Check sheet for the modelled part. Datum: model origin and axes. Units: mm. A direction names the side the tool comes from. Coordinates: 2 decimals unless noted, no trailing zeros. Order: outer loops, then holes, each group sorted by start corner. A loop starts at its lowest first (then second) coordinate and runs counter-clockwise, first axis right, second up.
from build123d import *

# Parameters (mm, degrees)
SKETCH2_R                           = 6.35
BOSS_EXTRUDE1_DEPTH                 = 12.7
FILLET3_R                           = 11.43
F_7_32_0_21875_DIAMETER_HOLE1_D     = 5.55625
F_7_32_0_21875_DIAMETER_HOLE1_DEPTH = 36.430734093
F_7_32_0_21875_DIAMETER_HOLE1_TIP   = 1.669265907


with BuildPart() as part:
    # Sketch2 → Boss-Extrude1 (new body)
    with BuildSketch(Plane.XY):
        Polygon((0, 0), (40.64, 0), (40.64, -10.16), (25.4, -10.16), (25.4, -22.86), (0, -22.86), align=None)
        with Locations((12.7, -11.43)):
            Circle(SKETCH2_R, mode=Mode.SUBTRACT)
    extrude(amount=BOSS_EXTRUDE1_DEPTH)

    # Fillet3
    fillet3_edges = [part.edges().sort_by_distance(p)[0] for p in [
        (0, -22.86, 6.35),
        (0, 0, 6.35),
    ]]
    fillet(fillet3_edges, radius=FILLET3_R - 0.0001)  # a hair under: the kernel refuses the full size

    # 7/32 (0.21875) Diameter Hole1
    with Locations(Plane(origin=(33.02, 0, 6.35), x_dir=(0, 0, 1), z_dir=(0, 1, 0))):
        with Locations((0, 0)):
            Hole(F_7_32_0_21875_DIAMETER_HOLE1_D / 2, depth=F_7_32_0_21875_DIAMETER_HOLE1_DEPTH)
            with Locations((0, 0, -(F_7_32_0_21875_DIAMETER_HOLE1_DEPTH + F_7_32_0_21875_DIAMETER_HOLE1_TIP / 2))):  # 118° drill point
                Cone(0, F_7_32_0_21875_DIAMETER_HOLE1_D / 2, F_7_32_0_21875_DIAMETER_HOLE1_TIP, mode=Mode.SUBTRACT)


solid = part.part
(1) Cross-section at A-A (x = 12.7). Enter the section's corners in (y, z).
Filled in:
outline: (-22.86, 0) - (-17.78, 0) - (-17.78, 12.7) - (-22.86, 12.7) - close; (-5.08, 0) - (0, 0) - (0, 12.7) - (-5.08, 12.7) - close
(2) Go/stop test with flat-tipped pins: P1, Ø4.5, axis at x = 33.02, z = 6.35, coming from the +Y side; P2, Ø1, axis at y = -19, z = 9.5, coming from the -X side; P3, Ø4, axis at x = 35, z = 7.5, coming from the -Y side; P4, Ø6, axis at y = -16, z = 9, coming from the -X side. Record where each tip stops, or that it passes through.
Filled in:
P1: passes through
P2: stops at x = 2.45
P3: stops at y = -10.16
P4: stops at x = 0.11
(3) Cross-section at B-B (y = -8). Enter the section's corners in (x, z), and give its area (3 significant figures).
Filled in:
outline: (0.53, 0) - (7.36, 0) - (7.36, 12.7) - (0.53, 12.7) - close; (18.04, 0) - (40.64, 0) - (40.64, 12.7) - (18.04, 12.7) - close; hole circle Ø5.56 at (33.02, 6.35)
area: 349 mm2
(4) Tool access check on faces 1 (the flat face through (25.4, -16, 6)), 2 (the cylindrical face through (3.259, -19.423, 6.439)). Record the directions out of +Z, -Z, +X, -X, +Y, -Y that give a thin tool (end or side, any length) a straight path to the whole face; none if there is none.
Filled in:
face 1: +Z, -Z, +X, -Y
face 2: +Z, -Z, -X, -Y
(5) Release check for a two-part mould opening along Y. For faces 3 (the flat face through (19, -22.86, 6)), 4 (the flat face through (21, -9, 12.7)), 5 (the cylindrical face through (3.437, -3.259, 6.439)), 6 (the cylindrical face through (8.02, -7.14, 6.26)) record: +Y half, -Y half, draft (parallel to the pull), parting line (faces both ways), or undercut.
Filled in:
face 3: -Y half
face 4: draft
face 5: +Y half
face 6: undercut
(6) Cross-section at C-C (z = 6.35). Count the separate pieces of the cut face and the enclosed holes in it, and give its area (3 significant figures).
Filled in:
separate pieces: 2
enclosed holes: 1
area: 496 mm2
(7) Thickness scan on probe 1 along Y at (x, z) = (12.7, 5); probe 2 along X at (y, z) = (-7.5, 6.35); probe 3 along X at (y, z) = (-6.75, 6.35). Record the ranges inside material, lowest first.
Filled in:
probe 1: y = -22.86 to -17.78, -5.08 to 0
probe 2: x = 0.7 to 7.71, 17.69 to 30.24, 35.8 to 40.64
probe 3: x = 1 to 8.41, 16.99 to 30.24, 35.8 to 40.64
